Input: part model. Units: mm. Frame: model coordinates. Coordinates: 2 decimals unless noted, no trailing zeros. Write each loop counter-clockwise with the first axis right and the second up, starting at its lowest first coordinate (ties: lowest second). Pieces come first, ordered by that corner, then holes.
1) Draft query along X for faces 1 (the conical face through (-150.2, -96, 1.7)), 2 (the flat face through (-147, -48, 2)), 3 (the flat face through (-10, -43, 0.6)). Return one class per face: pulls with the +X half, pulls with the -X half, needs draft (parallel to the pull), parting line crosses it, or undercut.
2) Section query A-A (z = 1.5). Output: boundary loops of the cut face in (x, y), then the cut area to 3 significant figures.
3) Pin query (flat end, axial travel): pin 1 Ø4 at (x, y) = (-4.5, -55.5) entering from -Z; pin 2 Ø1.2 at (x, z) = (-48, 1.5) entering from +Y; pin 3 Ø5 at (x, y) = (96, -46.5) entering from -Z. Return the tip coordinate at first contact, or that it passes through.
4) Line query: L1, parallel to X at y = -17, z = 1.6; L2, parallel to X at y = -83, z = 1.05; L3, parallel to Z at x = -91.5, y = -33.5. Output: solid intervals per line, ascending.
from build123d import *

# Parameters (mm, degrees)
BOSS_EXTRU_1_DEPTH      = 2
ENL_V_MAT_EXTRU_1_DEPTH = 1.4
ESQUISSE10_W            = 267.242852503
ESQUISSE10_H            = 8.975920375
BOSS_EXTRU_3_DEPTH      = 0.1
ESQUISSE11_W            = 12.5
ESQUISSE11_H            = 12.5
ENL_V_MAT_EXTRU_2_DEPTH = 0.1


with BuildPart() as part:
    # Esquisse1 → Boss.-Extru.1 (new body)
    with BuildSketch(Plane.XY):
        with BuildLine():
            Line((-154.451069542, 0), (-154.451069542, -92.3))
            ThreePointArc((-154.451069542, -92.3), (-152.107923791, -97.956854249), (-146.451069542, -100.3))
            Line((-146.451069542, -100.3), (129.548930458, -100.3))
            ThreePointArc((129.548930458, -100.3), (135.205784708, -97.956854249), (137.548930458, -92.3))
            Line((137.548930458, -92.3), (137.548930458, 0))
            Line((137.548930458, 0), (-154.451069542, 0))
        make_face()
    extrude(amount=BOSS_EXTRU_1_DEPTH)

    # Enlèvement de matière-Balayage3: sweep along a path in Esquisse3
    with BuildLine(Plane(origin=(0, 0, 0), x_dir=(-1, 0, 0), z_dir=(0, 0, -1))) as enl_vement_de_mati_re_balayage3_path:
        Line((154.451069542, 0.2), (154.451069542, -92.3))
        ThreePointArc((154.451069542, -92.3), (152.107923791, -97.956854249), (146.451069542, -100.3))
        Line((146.451069542, -100.3), (-129.548930458, -100.3))
        ThreePointArc((-129.548930458, -100.3), (-135.205784708, -97.956854249), (-137.548930458, -92.3))
        Line((-137.548930458, -92.3), (-137.548930458, 0.2))
    # Esquisse9 → Enlèvement de matière-Balayage3 (sweep, cut)
    with BuildSketch(Plane(origin=(0, 0, 0), x_dir=(1, 0, 0), z_dir=(0, 1, 0))):
        with BuildLine():
            Line((135.67035671, -1), (134.446277084, -2))
            Line((134.446277084, -2), (136.182569378, -2))
            Line((136.182569378, -2), (147.673144552, -2))
            Line((147.673144552, -2), (147.673144552, 0))
            Line((147.673144552, 0), (134.956411872, 0))
            add(Edge.make_bspline(
                [(134.956411872, 0), (135.206323755, -0.279338228), (135.44542126, -0.617312994), (135.67035671, -1)],
                knots=[0, 0, 0, 0, 0.17887146, 0.17887146, 0.17887146, 0.17887146], degree=3))
        make_face()
    sweep(path=enl_vement_de_mati_re_balayage3_path.line, mode=Mode.SUBTRACT)

    # Esquisse5 → Enlèv. mat.-Extru.1 (cut)
    with BuildSketch(Plane.XY.offset(2)):
        with BuildLine():
            Line((124.926952048, -84.47802159), (124.926952048, 0))
            Line((124.926952048, 0), (-141.829091132, 0))
            Line((-141.829091132, 0), (-141.829091132, -84.47802159))
            ThreePointArc((-141.829091132, -84.47802159), (-140.950411475, -86.599341934), (-138.829091132, -87.47802159))
            Line((-138.829091132, -87.47802159), (121.926952048, -87.47802159))
            ThreePointArc((121.926952048, -87.47802159), (124.048272392, -86.599341934), (124.926952048, -84.47802159))
        make_face()
        with BuildLine():
            Line((-142.072495793, -88.221426251), (125.17035671, -88.221426251))
            Line((125.17035671, -88.221426251), (125.17035671, 0))
            Line((125.17035671, 0), (124.926952048, 0))
            Line((124.926952048, 0), (124.926952048, -84.47802159))
            ThreePointArc((124.926952048, -84.47802159), (124.048272392, -86.599341934), (121.926952048, -87.47802159))
            Line((121.926952048, -87.47802159), (-138.829091132, -87.47802159))
            ThreePointArc((-138.829091132, -87.47802159), (-140.950411475, -86.599341934), (-141.829091132, -84.47802159))
            Line((-141.829091132, -84.47802159), (-141.829091132, 0))
            Line((-141.829091132, 0), (-142.072495793, 0))
            Line((-142.072495793, 0), (-142.072495793, -88.221426251))
        make_face()
    extrude(amount=-ENL_V_MAT_EXTRU_1_DEPTH, mode=Mode.SUBTRACT)

    # Esquisse10 → Boss.-Extru.3 (add)
    with BuildSketch(Plane.XY.offset(2)):
        with Locations((-8.451069541, -92.709386439)):
            Rectangle(ESQUISSE10_W, ESQUISSE10_H)
    extrude(amount=BOSS_EXTRU_3_DEPTH)

    # Esquisse11 → Enlèv. mat.-Extru.2 (cut)
    with BuildSketch(Plane(origin=(0, 0, 0), x_dir=(-1, 0, 0), z_dir=(0, 0, -1))):
        with Locations((1.501069542, -55.671426251)):
            Rectangle(ESQUISSE11_W, ESQUISSE11_H)
        with Locations((1.501069542, -41.771426251)):
            Rectangle(ESQUISSE11_W, ESQUISSE11_H)
        with Locations((15.401069542, -41.771426251)):
            Rectangle(ESQUISSE11_W, ESQUISSE11_H)
        with Locations((15.401069542, -55.671426251)):
            Rectangle(ESQUISSE11_W, ESQUISSE11_H)
    extrude(amount=-ENL_V_MAT_EXTRU_2_DEPTH, mode=Mode.SUBTRACT)


solid = part.part
Answer:
1. face 1: pulls with the -X half
1. face 2: needs draft
1. face 3: undercut
2. outline: (-151.96, -92.3) arc R5.51 ccw to (-146.45, -97.81) - (129.55, -97.81) arc R5.51 ccw to (135.06, -92.3) - (135.06, 0) - (125.17, 0) - (125.17, -88.22) - (-142.07, -88.22) - (-142.07, 0) - (-151.96, 0) - close
2. area: 4,480 mm2
3. pin 1: stops at z = 0.1
3. pin 2: stops at y = -88.22
3. pin 3: stops at z = 0
4. L1: x = -151.84 to -142.07, 125.17 to 134.94
4. L2: x = -152.51 to -142.07, 125.17 to 135.61
4. L3: z = 0 to 0.6
